```python
from build123d import *

# Parameters (mm, degrees)
BOSS_EXTRUDE1_DEPTH = 10
SKETCH3_R           = 3.5
SKETCH3_R_2         = 2
CUT_EXTRUDE1_DEPTH  = 30


with BuildPart() as part:
    # Sketch2 → Boss-Extrude1 (new body)
    with BuildSketch(Plane(origin=(0, 0, 0), x_dir=(1, 0, 0), z_dir=(0, 1, 0))):
        Polygon((0, 0), (15, 0), (25, 15), (40, 15), (40, 13), (27, 13), (17, -2), (0, -2), align=None)
    extrude(amount=BOSS_EXTRUDE1_DEPTH)

    # Sketch3 → Cut-Extrude1 (cut)
    with BuildSketch(Plane.XY.offset(2)):
        with Locations((8.5, 5)):
            Circle(SKETCH3_R)
        with Locations((33.5, 5)):
            Circle(SKETCH3_R_2)
    extrude(amount=-CUT_EXTRUDE1_DEPTH, mode=Mode.SUBTRACT)


solid = part.part
```
Verification items for the finished model (mm, model axes). A direction names the side the tool comes from. Coordinates: 2 decimals unless noted, no trailing zeros. Loops run counter-clockwise (first coordinate to the right, second up) from the corner with the lowest first, then second, coordinate; pieces in that order, holes last. Notation, with made-up numbers: (-39.75, 81.25) - (-23.75, 81.25) arc R12 cw to (-23.75, 100.25) - close; hole circle Ø1 at (59.5, 26). An arc over 180 degrees is marked (long way). Return JSON: item names as keys, results as strings.
1. Mould release check, pull along Y, two halves, no side actions. Record for faces 1 (the flat face through (20, 0, -7)), 2 (the cylindrical face through (5, 5, 1)), 3 (the flat face through (31, 5, -15)): +Y half, -Y half, draft (parallel to the pull), parting line (faces both ways), or undercut.
Established:
{"face 1": "-Y half", "face 2": "undercut", "face 3": "draft"}
2. Tool access check on faces 4 (the flat face through (33.6, 2.7, -13)), 5 (the flat face through (4, 5, 0)), 6 (the flat face through (4.8, 4.9, 2)). Record the directions out of +Z, -Z, +X, -X, +Y, -Y that give a thin tool (end or side, any length) a straight path to the whole face; none if there is none.
Established:
{"face 4": "+Z, +X, +Y, -Y", "face 5": "-Z, -X, +Y, -Y", "face 6": "+Z, +X, -X, +Y, -Y"}
3. Go/stop test with flat-tipped pins: pin 1 (5 mm diameter, centred on y = 3.5, z = -12.5, fed in from -X); pin 2 (5.5 mm diameter, centred on x = 8.5, y = 5, fed in from +Z); pin 3 (3 mm diameter, centred on x = 34.5, y = 6.5, fed in from +Z); pin 4 (1 mm diameter, centred on y = 4, z = -7.5, fed in from +X). Record where each tip stops, or that it passes through.
Established:
{"pin 1": "stops at x = 21.67", "pin 2": "passes through", "pin 3": "stops at z = -13", "pin 4": "stops at x = 23.67"}
4. Section check C-C, the plane y = 9.25. Record the boundary of the cut face in (x, z), then the cut area to 3 significant figures.
Established:
{"outline": "(0, 0) - (15, 0) - (25, -15) - (40, -15) - (40, -13) - (27, -13) - (17, 2) - (0, 2) - close", "area": "110 mm2"}
5. Section check A-A, the plane y = 5. Record the boundary of the cut face in (x, z).
Established:
{"outline": "(0, 0) - (5, 0) - (5, 2) - (0, 2) - close; (12, 0) - (15, 0) - (25, -15) - (31.5, -15) - (31.5, -13) - (27, -13) - (17, 2) - (12, 2) - close; (35.5, -15) - (40, -15) - (40, -13) - (35.5, -13) - close"}
6. Section check B-B, the plane x = 33.5. Record the boundary of the cut face in (y, z), then the cut area to 3 significant figures.
Established:
{"outline": "(0, -15) - (3, -15) - (3, -13) - (0, -13) - close; (7, -15) - (10, -15) - (10, -13) - (7, -13) - close", "area": "12.0 mm2"}
7. Section check D-D, the plane x = 8.5. Record the boundary of the cut face in (y, z), then the cut area to 3 significant figures.
Established:
{"outline": "(0, 0) - (1.5, 0) - (1.5, 2) - (0, 2) - close; (8.5, 0) - (10, 0) - (10, 2) - (8.5, 2) - close", "area": "6.00 mm2"}
8. Thickness scan on L1, parallel to Y at x = 33.5, z = -13.7; L2, parallel to Z at x = 7, y = 1; L3, parallel to Z at x = 38, y = 7.25. Record the ranges inside material, lowest first.
Established:
{"L1": "y = 0 to 3, 7 to 10", "L2": "z = 0 to 2", "L3": "z = -15 to -13"}
